```python
from build123d import *

# Parameters (mm, degrees)
SKETCH1_W           = 7
SKETCH1_H           = 3
SKETCH1_W_2         = 17
SKETCH1_H_2         = 3.275
BOSS_EXTRUDE1_DEPTH = 15


with BuildPart() as part:
    # Sketch1 → Boss-Extrude1 (new body)
    with BuildSketch(Plane.XY):
        with Locations((12, 20.325)):
            Rectangle(SKETCH1_W, SKETCH1_H)
        with Locations((0, 20.325)):
            Rectangle(SKETCH1_W_2, SKETCH1_H)
        with Locations((-12, 20.325)):
            Rectangle(SKETCH1_W, SKETCH1_H)
        with Locations((0, 17.1875)):
            Rectangle(SKETCH1_W_2, SKETCH1_H_2)
        with BuildLine():
            ThreePointArc((-15.5, 0), (0, 15.5), (15.5, 0))
            Line((15.5, 0), (15.5, 15.55))
            Line((15.5, 15.55), (8.5, 15.55))
            Line((8.5, 15.55), (-8.5, 15.55))
            Line((-8.5, 15.55), (-15.5, 15.55))
            Line((-15.5, 15.55), (-15.5, 0))
        make_face()
        with BuildLine():
            ThreePointArc((-12.575, 0), (0, 12.575), (12.575, 0))
            Line((12.575, 0), (15.5, 0))
            ThreePointArc((15.5, 0), (0, 15.5), (-15.5, 0))
            Line((-15.5, 0), (-12.575, 0))
        make_face()
        with BuildLine():
            Line((15.5, 0), (12.575, 0))
            ThreePointArc((12.575, 0), (0, -12.575), (-12.575, 0))
            Line((-12.575, 0), (-15.5, 0))
            ThreePointArc((-15.5, 0), (0, -15.5), (15.5, 0))
        make_face()
    extrude(amount=BOSS_EXTRUDE1_DEPTH)


solid = part.part
```
Read the model definition and answer for the solid it produces. Units are mm, in the model's axes. A direction names the side the tool comes from. Give positions to 0.01 mm unless a question says otherwise; leave off trailing zeros. Write each loop counter-clockwise with the first axis right and the second up, starting at its lowest first coordinate (ties: lowest second). Pieces come first, ordered by that corner, then holes. Notation, with made-up numbers: (79, -35) - (106, -35) arc R24 cw to (106, -21) - close; hole circle Ø4 at (-30.75, -20.5). An arc over 180 degrees is marked (long way). Write item = value, one per line. Start each with the question number.
Item 1: Find section A-A (x = 0). Give the vertices of the cut face in (y, z) (3 decimals).
Item 2: Find section C-C (y = 7). Give the vertices of the cut face in (x, z).
Item 3: Find the intervals of material crossed by probe 1 along Y at (x, z) = (0, 11.75) (3 decimals); probe 2 along Y at (x, z) = (-9, 6.5) (3 decimals); probe 3 along X at (y, z) = (18.5, 7), in increasing order. Write a range as [from, to].
Item 4: Find section D-D (y = 18). Give the vertices of the cut face in (x, z).
Item 5: A tool of negligible diameter and unlimited length cuts with its end or side. For faces 1 (the flat face through (-12, 15.55, 7)), 2 (the flat face through (-7, 12, 15)), 3 (the flat face through (12, 15.55, 7)), from which of +Z, -Z, +X, -X, +Y, -Y can it reach the whole face along a straight path? Write none if from no direction.
Item 6: The mould has two halves that part along Y. Classify faces 4 (the flat face through (0, 21.825, 7)), 5 (the flat face through (12, 18.825, 7)), 6 (the flat face through (-15.5, 8, 7)), 7 (the cylindrical face through (-0.341, -15.496, 7.395)): +Y half, -Y half, draft (parallel to the pull), parting line (faces both ways), or undercut.
Item 7: Each of these flat-tipped pins is pushed along its axis until it touches: P1, Ø1.5, axis at y = 17.5, z = 7, coming from the +X side; P2, Ø5.5, axis at x = 13.5, z = 4.5, coming from the -Y side; P3, Ø2, axis at y = -2.5, z = 6, coming from the +X side; P4, Ø12, axis at x = 11.5, y = 16, coming from the +Z side. Where does it stop, or does it pass through?
Item 8: Find section B-B (z = 8.75). Give the vertices of the cut face in (x, y) (3 decimals).
Response:
q1.outline = (-15.5, 0) - (-12.575, 0) - (-12.575, 15) - (-15.5, 15) - close; (12.575, 0) - (21.825, 0) - (21.825, 15) - (12.575, 15) - close
q2.outline = (-15.5, 0) - (-10.45, 0) - (-10.45, 15) - (-15.5, 15) - close; (10.45, 0) - (15.5, 0) - (15.5, 15) - (10.45, 15) - close
q3.probe_1 = [-15.5, -12.575], [12.575, 21.825]
q3.probe_2 = [-12.619, -8.782], [8.782, 15.55], [18.825, 21.825]
q3.probe_3 = [-8.5, 8.5]
q4.outline = (-8.5, 0) - (8.5, 0) - (8.5, 15) - (-8.5, 15) - close
q5.face_1 = +Z, -Z, -X
q5.face_2 = +Z, +X, -X, +Y, -Y
q5.face_3 = +Z, -Z, +X
q6.face_4 = +Y half
q6.face_5 = undercut
q6.face_6 = draft
q6.face_7 = -Y half
q7.P1 = 8.5
q7.P2 = -11.17
q7.P3 = 15.43
q7.P4 = 15
q8.outline = (-15.5, 0) arc R15.5 ccw to (15.5, 0) - (15.5, 15.55) - (8.5, 15.55) - (8.5, 18.825) - (15.5, 18.825) - (15.5, 21.825) - (-15.5, 21.825) - (-15.5, 18.825) - (-8.5, 18.825) - (-8.5, 15.55) - (-15.5, 15.55) - close; hole circle Ø25.15 at (0, 0)
